```python
from build123d import *

# Parameters (mm, degrees)
SKETCH1_R           = 4
SKETCH1_R_2         = 1.6
SKETCH1_R_3         = 1.8
SKETCH1_R_4         = 1.3
BOSS_EXTRUDE1_DEPTH = 5.5
SKETCH2_R           = 2.8
CUT_EXTRUDE1_DEPTH  = 3.2
CHAMFER1_SIZE       = 0.2


with BuildPart() as part:
    # Sketch1 → Boss-Extrude1 (new body)
    # profile 1 of 7: a face of its own
    with BuildSketch(Plane.XY):
        with BuildLine():
            Line((30.355028895, 9.984213157), (-20.144971105, 14.484213157))
            ThreePointArc((-20.144971105, 14.484213157), (-17.548719297, 13.199989298), (-16.5, 10.5))
            ThreePointArc((-16.5, 10.5), (-22.638997252, 7.119956989), (-22.212345379, 14.114951356))
            Line((-22.212345379, 14.114951356), (-31.712345379, 9.614951356))
            ThreePointArc((-31.712345379, 9.614951356), (-27.861002748, 9.380043011), (-26, 6))
            ThreePointArc((-26, 6), (-27.651511703, 2.762006375), (-31.242301359, 2.197804932))
            Line((-31.242301359, 2.197804932), (19.257698641, -14.302195068))
            ThreePointArc((19.257698641, -14.302195068), (18.151511703, -7.262006375), (24.5, -10.5))
            ThreePointArc((24.5, -10.5), (24.364321371, -11.532966769), (23.966489827, -12.495857779))
            Line((23.966489827, -12.495857779), (33.466489827, 4.004142221))
            ThreePointArc((33.466489827, 4.004142221), (26.451575922, 4.153737137), (30.355028895, 9.984213157))
        make_face()
    # profile 2 of 7: a face of its own
    with BuildSketch(Plane.XY):
        with Locations((-30, 6)):
            Circle(SKETCH1_R)
        with Locations((-30, 6)):
            Circle(SKETCH1_R_2, mode=Mode.SUBTRACT)
    # profile 3 of 7: a face of its own
    with BuildSketch(Plane.XY):
        with Locations((-20.5, 10.5)):
            Circle(SKETCH1_R)
        with Locations((-20.5, 10.5)):
            Circle(SKETCH1_R_3, mode=Mode.SUBTRACT)
    # profile 4 of 7: a face of its own
    with BuildSketch(Plane.XY):
        with Locations((30, 6)):
            Circle(SKETCH1_R)
        with Locations((30, 6)):
            Circle(SKETCH1_R_2, mode=Mode.SUBTRACT)
    # profile 5 of 7: a face of its own
    with BuildSketch(Plane.XY):
        with Locations((20.5, -10.5)):
            Circle(SKETCH1_R)
        with Locations((20.5, -10.5)):
            Circle(SKETCH1_R_3, mode=Mode.SUBTRACT)
    # profile 6 of 7: a face of its own
    with BuildSketch(Plane.XY):
        with Locations((-20.5, 10.5)):
            Circle(SKETCH1_R_3)
        with Locations((-20.5, 10.5)):
            Circle(SKETCH1_R_4, mode=Mode.SUBTRACT)
    # profile 7 of 7: a face of its own
    with BuildSketch(Plane.XY):
        with Locations((20.5, -10.5)):
            Circle(SKETCH1_R_3)
        with Locations((20.5, -10.5)):
            Circle(SKETCH1_R_4, mode=Mode.SUBTRACT)
    extrude(amount=BOSS_EXTRUDE1_DEPTH)

    # Sketch2 → Cut-Extrude1 (cut)
    with BuildSketch(Plane.XY):
        with Locations((-30, 6)):
            Circle(SKETCH2_R)
        with Locations((30, 6)):
            Circle(SKETCH2_R)
    extrude(amount=CUT_EXTRUDE1_DEPTH, mode=Mode.SUBTRACT)

    # Chamfer1
    chamfer1_edges = [part.edges().sort_by_distance(p)[0] for p in [
        (33.548424078, 7.846262863, 5.5),
        (-21.8, 10.5, 0),
        (19.2, -10.5, 0),
        (21.932643426, -14.234639583, 0),
        (-5.992301359, -6.052195068, 0),
        (-33.991991934, 5.747017002, 0),
        (-26.962345379, 11.864951356, 0),
        (-21.203324661, 14.437681351, 0),
        (5.105028895, 12.234213157, 0),
        (5.105028895, 12.234213157, 5.5),
        (33.548424078, 7.846262863, 0),
        (28.716489827, -4.245857779, 0),
        (-21.203324661, 14.437681351, 5.5),
        (-26.962345379, 11.864951356, 5.5),
        (-33.991991934, 5.747017002, 5.5),
        (-5.992301359, -6.052195068, 5.5),
        (21.932643426, -14.234639583, 5.5),
        (-31.6, 6, 5.5),
        (28.4, 6, 5.5),
        (-32.8, 6, 0),
        (19.2, -10.5, 5.5),
        (27.2, 6, 0),
        (-21.8, 10.5, 5.5),
        (28.716489827, -4.245857779, 5.5),
    ]]
    chamfer(chamfer1_edges, length=CHAMFER1_SIZE)


solid = part.part
```
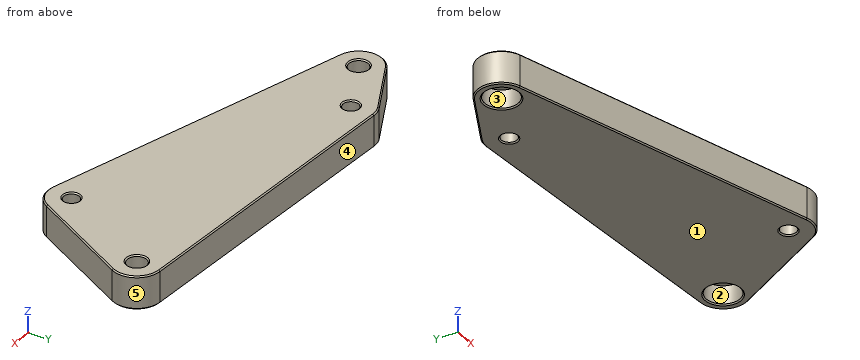
Input: part model. Units: mm. Frame: model coordinates. Face numbers are marked on the shaded views. A direction names the side the tool comes from. Coordinates: 2 decimals unless noted, no trailing zeros. Loops run counter-clockwise (first coordinate to the right, second up) from the corner with the lowest first, then second, coordinate; pieces in that order, holes last. Notation, with made-up numbers: M 17,39.5 L 25,39.5 A20 cw 25,48.5 Z; hole C 30.25,9.5 d4. An arc over 180 degrees is marked long. Use a Markdown table: item, result. Add a question column.
1) Set-up query: the marked faces 1 and 2. Return all of +Z, -Z, +X, -X, +Y, -Y with unobstructed straight access to the full face (end or side cutting, diameter ignored); none if empty.
2) Line query: L1, parallel to X at y = 6, z = 4; L2, parallel to X at y = 4, z = 1.95; L3, parallel to Y at x = -30, z = 4.1. Output: solid intervals per line, ascending. Write a range as from..to.
3) Section B-B, the plane x = 20.5. Return the cut outline in (y, z), plus the area to 3 significant figures.
4) Pin query (flat end, axial travel): P1, Ø1, axis at x = -2, z = 3.5, coming from the +Y side; P2, Ø3, axis at y = 3.5, z = 1, coming from the +X side; P3, Ø4, axis at x = 30, y = 6, coming from the -Z side; P4, Ø2.5, axis at x = -20.5, y = 10.5, coming from the +Z side. Return the tip coordinate at first contact, or that it passes through.
5) Section D-D, the plane y = -10.5. Return the cut outline in (x, z), plus the area to 3 significant figures.
6) Section C-C, the plane y = 6. Give the number of separate pieces and of enclosed holes in the cut face, plus the area to 3 significant figures.
7) Section A-A, the plane z = 3.95. Return the cut outline in (x, y).
8) Draft query along Y for the marked faces 3, 4 and 5. Return one class per face: +Y half, -Y half, draft (parallel to the pull), parting line (faces both ways), or undercut.
Answer below:
| question | item | result |
|---|---|---|
| 1 | face 1 | -Z, +X, -X, +Y, -Y |
| 1 | face 2 | -Z |
| 2 | L1 | -34..-31.6, -28.4..28.4, 31.6..34 |
| 2 | L2 | -33.46..-31.96, -28.04..28.04, 31.96..33.46 |
| 2 | L3 | 1.79..4.4, 7.6..10.43 |
| 3 | outline | M -14.5,0.2 L -14.3,0 L -12,0 L -11.8,0.2 L -11.8,5.3 L -12,5.5 L -14.3,5.5 L -14.5,5.3 Z; M -9.2,0.2 L -9,0 L 10.66,0 L 10.86,0.2 L 10.86,5.3 L 10.66,5.5 L -9,5.5 L -9.2,5.3 Z |
| 3 | area | 125 mm2 |
| 4 | P1 | y = 12.91 |
| 4 | P2 | x = 33.87 |
| 4 | P3 | z = 3.2 |
| 4 | P4 | through |
| 5 | outline | M 7.62,0.2 L 8.26,0 L 19,0 L 19.2,0.2 L 19.2,5.3 L 19,5.5 L 8.26,5.5 L 7.62,5.3 Z; M 21.8,0.2 L 22,0 L 24.88,0 L 25.12,0.2 L 25.12,5.3 L 24.88,5.5 L 22,5.5 L 21.8,5.3 Z |
| 5 | area | 81.7 mm2 |
| 6 | separate pieces | 3 |
| 6 | enclosed holes | 0 |
| 6 | area | 323 mm2 |
| 7 | outline | M -31.71,9.61 A4 ccw -31.24,2.2 L 19.26,-14.3 A4 ccw 23.97,-12.5 L 33.47,4 A4 ccw 30.36,9.98 L -20.14,14.48 A4 ccw -22.21,14.11 Z; hole C -30,6 d3.2; hole C -20.5,10.5 d2.6; hole C 20.5,-10.5 d2.6; hole C 30,6 d3.2 |
| 8 | face 3 | undercut |
| 8 | face 4 | +Y half |
| 8 | face 5 | parting line |
